from build123d import *

# Parameters (mm, degrees)
SKETCH1_W           = 177.8
SKETCH1_H           = 114.3
SKETCH1_W_2         = 165.1
SKETCH1_H_2         = 16.134929366
BOSS_EXTRUDE1_DEPTH = 4.7625
CUT_EXTRUDE1_DEPTH  = 5.7625
SKETCH4_R           = 2.38125
CUT_EXTRUDE2_DEPTH  = 5.7625
SKETCH7_W           = 12.7
SKETCH7_H           = 4.7625
BOSS_EXTRUDE2_DEPTH = 4.7625
SKETCH8_W           = 12.7
SKETCH8_H           = 4.7625
BOSS_EXTRUDE3_DEPTH = 4.7625


with BuildPart() as part:
    # Sketch1 → Boss-Extrude1 (new body)
    with BuildSketch(Plane(origin=(0, 0, 0), x_dir=(1, 0, 0), z_dir=(0, 1, 0))):
        Rectangle(SKETCH1_W, SKETCH1_H)
        with BuildLine():
            Line((-82.55, -25.4), (-82.55, -20.767464683))
            Line((-82.55, -20.767464683), (82.55, -20.767464683))
            Line((82.55, -20.767464683), (82.55, -25.4))
            ThreePointArc((82.55, -25.4), (64.589487758, -32.839487758), (57.15, -50.8))
            Line((57.15, -50.8), (-57.15, -50.8))
            ThreePointArc((-57.15, -50.8), (-64.589487758, -32.839487758), (-82.55, -25.4))
        make_face(mode=Mode.SUBTRACT)
        Rectangle(SKETCH1_W_2, SKETCH1_H_2, mode=Mode.SUBTRACT)
        with BuildLine():
            Line((82.55, 20.767464683), (-82.55, 20.767464683))
            Line((-82.55, 20.767464683), (-82.55, 25.4))
            ThreePointArc((-82.55, 25.4), (-64.589487758, 32.839487758), (-57.15, 50.8))
            Line((-57.15, 50.8), (57.15, 50.8))
            ThreePointArc((57.15, 50.8), (64.589487758, 32.839487758), (82.55, 25.4))
            Line((82.55, 25.4), (82.55, 20.767464683))
        make_face(mode=Mode.SUBTRACT)
    extrude(amount=BOSS_EXTRUDE1_DEPTH)

    # Sketch3 → Cut-Extrude1 (cut, through all)
    with BuildSketch(Plane(origin=(0, 4.7625, 0), x_dir=(1, 0, 0), z_dir=(0, 1, 0))):
        with BuildLine():
            Line((-76.2, 16.004964683), (76.2, 16.004964683))
            ThreePointArc((76.2, 16.004964683), (77.7875, 14.417464683), (76.2, 12.829964683))
            Line((76.2, 12.829964683), (-76.2, 12.829964683))
            ThreePointArc((-76.2, 12.829964683), (-77.7875, 14.417464683), (-76.2, 16.004964683))
        make_face()
        with BuildLine():
            Line((-76.2, -16.004964683), (76.2, -16.004964683))
            ThreePointArc((76.2, -16.004964683), (77.7875, -14.417464683), (76.2, -12.829964683))
            Line((76.2, -12.829964683), (-76.2, -12.829964683))
            ThreePointArc((-76.2, -12.829964683), (-77.7875, -14.417464683), (-76.2, -16.004964683))
        make_face()
    extrude(amount=-CUT_EXTRUDE1_DEPTH, mode=Mode.SUBTRACT)

    # Sketch4 → Cut-Extrude2 (cut, through all)
    with BuildSketch(Plane(origin=(0, 4.7625, 0), x_dir=(1, 0, 0), z_dir=(0, 1, 0))):
        with Locations((-76.2, 39.37)):
            Circle(SKETCH4_R)
        with Locations((-76.2, -39.37)):
            Circle(SKETCH4_R)
        with Locations((76.2, -39.37)):
            Circle(SKETCH4_R)
        with Locations((76.2, 39.37)):
            Circle(SKETCH4_R)
    extrude(amount=-CUT_EXTRUDE2_DEPTH, mode=Mode.SUBTRACT)

    # Sketch7 → Boss-Extrude2 (add)
    with BuildSketch(Plane(origin=(88.9, 0, 0), x_dir=(0, 0, -1), z_dir=(1, 0, 0))):
        with Locations((-38.1, 2.38125)):
            Rectangle(SKETCH7_W, SKETCH7_H)
        with Locations((12.7, 2.38125)):
            Rectangle(SKETCH7_W, SKETCH7_H)
    extrude(amount=BOSS_EXTRUDE2_DEPTH)

    # Sketch8 → Boss-Extrude3 (add)
    with BuildSketch(Plane.ZY.offset(88.9)):
        with Locations((-38.1, 2.38125)):
            Rectangle(SKETCH8_W, SKETCH8_H)
        with Locations((12.7, 2.38125)):
            Rectangle(SKETCH8_W, SKETCH8_H)
    extrude(amount=BOSS_EXTRUDE3_DEPTH)


solid = part.part
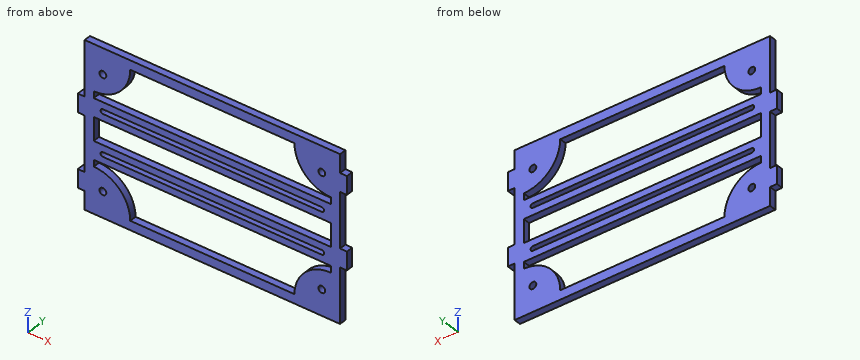
Source: CAD feature listing. Evaluate the final solid. Frame: model axes, mm. Round coordinates to 2 decimals unless told otherwise and drop trailing zeros. Order: outer loops, then holes, each group sorted by start corner. A loop starts at its lowest first (then second) coordinate and runs counter-clockwise, first axis right, second up. Notation, with made-up numbers: (85, 67) - (122, 67) arc R23 cw to (122, 80) - close; hole circle Ø10 at (77.25, -36.5). An arc over 180 degrees is marked (long way). Use a Markdown table: item, result. Add a question column.
1. First-contact query: pin 1 (2.5 mm diameter, centred on y = 2, z = -53.5, fed in from -X); pin 2 (4 mm diameter, centred on x = 76.2, z = 39.37, fed in from -Y); pin 3 (2.5 mm diameter, centred on x = -91, y = 3.5, fed in from +Z). Flat tips, straight axial feed; report the tip coordinate or a pass-through.
2. Line query: probe 1 along Z at (x, y) = (22, 3.6); probe 2 along Z at (x, y) = (-78, 3.3); probe 3 along X at (y, z) = (2.7, 38). Output: solid intervals per line, ascending.
3. Section query B-B (x = -7.5). Return the cut outline in (y, z), then the cut area to 3 significant figures.
4. Section query A-A (z = -23). Return the cut outline in (x, y), then the cut area to 3 significant figures.
5. Section query D-D (y = 1.2). Give the number of separate pieces and of enclosed holes in the cut face, then the cut area to 3 significant figures.
6. Section query C-C (z = 39.37). Return the cut outline in (x, y), then the cut area to 3 significant figures.
Derived:
| question | item | result |
|---|---|---|
| 1 | pin 1 | x = -88.9 |
| 1 | pin 2 | through |
| 1 | pin 3 | z = 19.05 |
| 2 | probe 1 | -57.15 to -50.8, -20.77 to -16, -12.83 to -8.07, 8.07 to 12.83, 16 to 20.77, 50.8 to 57.15 |
| 2 | probe 2 | -57.15 to -40.93, -37.81 to -25.81, -20.77 to -8.07, 8.07 to 20.77, 25.81 to 37.81, 40.93 to 57.15 |
| 2 | probe 3 | -88.9 to -78.15, -74.25 to -60.61, 60.61 to 74.25, 78.15 to 93.66 |
| 3 | outline | (0, -57.15) - (4.76, -57.15) - (4.76, -50.8) - (0, -50.8) - close; (0, -20.77) - (4.76, -20.77) - (4.76, -16) - (0, -16) - close; (0, -12.83) - (4.76, -12.83) - (4.76, -8.07) - (0, -8.07) - close; (0, 8.07) - (4.76, 8.07) - (4.76, 12.83) - (0, 12.83) - close; (0, 16) - (4.76, 16) - (4.76, 20.77) - (0, 20.77) - close; (0, 50.8) - (4.76, 50.8) - (4.76, 57.15) - (0, 57.15) - close |
| 3 | area | 151 mm2 |
| 4 | outline | (-88.9, 0) - (-82.55, 0) - (-82.55, 4.76) - (-88.9, 4.76) - close; (82.55, 0) - (88.9, 0) - (88.9, 4.76) - (82.55, 4.76) - close |
| 4 | area | 60.5 mm2 |
| 5 | separate pieces | 1 |
| 5 | enclosed holes | 9 |
| 5 | area | 8,960 mm2 |
| 6 | outline | (-88.9, 0) - (-78.58, 0) - (-78.58, 4.76) - (-88.9, 4.76) - close; (-73.82, 0) - (-59.87, 0) - (-59.87, 4.76) - (-73.82, 4.76) - close; (59.87, 0) - (73.82, 0) - (73.82, 4.76) - (59.87, 4.76) - close; (78.58, 0) - (93.66, 0) - (93.66, 4.76) - (78.58, 4.76) - close |
| 6 | area | 254 mm2 |
